from build123d import *

# Parameters (mm, degrees)
SKETCH1_W               = 166
SKETCH1_H               = 116
BOX_SOLID_DEPTH         = 53
BOX_CAVITY_START        = 3
SKETCH2_W               = 160
SKETCH2_H               = 110
BOX_CAVITY_DEPTH        = 53
LID_SCREW_COLUMNS_START = 3
SKETCH3_R               = 3.5
LID_SCREW_COLUMNS_DEPTH = 50
LID_SCREW_HOLES_START   = 53
SKETCH4_R               = 1.25
LID_SCREW_HOLES_DEPTH   = 10
RELAY_BOSSES_START      = 3
SKETCH5_R               = 3.25
RELAY_BOSSES_DEPTH      = 5
RELAY_BOSS_HOLES_START  = 8
SKETCH6_R               = 1.25
RELAY_BOSS_HOLES_DEPTH  = 5
BOARD_PADS_START        = 3
SKETCH7_R               = 2.5
BOARD_PADS_DEPTH        = 5
CABLE_GLAND_HOLES_START = 54
SKETCH8_R               = 6.25
CABLE_GLAND_HOLES_DEPTH = 5
VENT_SLOTS_START        = -84
SKETCH9_W               = 3
SKETCH9_H               = 26
VENT_SLOTS_DEPTH        = 5
SKETCH10_R              = 5
LEG_SOCKETS_DEPTH       = 2


with BuildPart() as part:
    # Sketch1 → Box_Solid (new body)
    with BuildSketch(Plane(origin=(0, 0, 0), x_dir=(1, 0, 0), z_dir=(0, 1, 0))):
        Rectangle(SKETCH1_W, SKETCH1_H)
    extrude(amount=BOX_SOLID_DEPTH)

    # Sketch2 → Box_Cavity (cut)
    with BuildSketch(Plane(origin=(0, 0, 0), x_dir=(1, 0, 0), z_dir=(0, 1, 0)).offset(BOX_CAVITY_START)):
        Rectangle(SKETCH2_W, SKETCH2_H)
    extrude(amount=BOX_CAVITY_DEPTH, mode=Mode.SUBTRACT)

    # Sketch3 → Lid_Screw_Columns (add)
    with BuildSketch(Plane(origin=(0, 0, 0), x_dir=(1, 0, 0), z_dir=(0, 1, 0)).offset(LID_SCREW_COLUMNS_START)):
        with Locations((-77, 52)):
            Circle(SKETCH3_R)
        with Locations((-77, -52)):
            Circle(SKETCH3_R)
        with Locations((77, 52)):
            Circle(SKETCH3_R)
        with Locations((77, -52)):
            Circle(SKETCH3_R)
    extrude(amount=LID_SCREW_COLUMNS_DEPTH)

    # Sketch4 → Lid_Screw_Holes (cut)
    with BuildSketch(Plane(origin=(0, 0, 0), x_dir=(1, 0, 0), z_dir=(0, 1, 0)).offset(LID_SCREW_HOLES_START)):
        with Locations(Location((-77, 52, 0), (0, 0, 270))):
            Circle(SKETCH4_R)
        with Locations(Location((-77, -52, 0), (0, 0, 270))):
            Circle(SKETCH4_R)
        with Locations(Location((77, 52, 0), (0, 0, 270))):
            Circle(SKETCH4_R)
        with Locations(Location((77, -52, 0), (0, 0, 270))):
            Circle(SKETCH4_R)
    extrude(amount=-LID_SCREW_HOLES_DEPTH, mode=Mode.SUBTRACT)

    # Sketch5 → Relay_Bosses (add)
    with BuildSketch(Plane(origin=(0, 0, 0), x_dir=(1, 0, 0), z_dir=(0, 1, 0)).offset(RELAY_BOSSES_START)):
        with Locations(Location((-68.5, 44.5, 0), (0, 0, 90))):
            Circle(SKETCH5_R)
        with Locations(Location((-68.5, -4.5, 0), (0, 0, 90))):
            Circle(SKETCH5_R)
        with Locations(Location((0.5, 44.5, 0), (0, 0, 90))):
            Circle(SKETCH5_R)
        with Locations(Location((0.5, -4.5, 0), (0, 0, 90))):
            Circle(SKETCH5_R)
    extrude(amount=RELAY_BOSSES_DEPTH)

    # Sketch6 → Relay_Boss_Holes (cut)
    with BuildSketch(Plane(origin=(0, 0, 0), x_dir=(1, 0, 0), z_dir=(0, 1, 0)).offset(RELAY_BOSS_HOLES_START)):
        with Locations(Location((-68.5, 44.5, 0), (0, 0, 270))):
            Circle(SKETCH6_R)
        with Locations(Location((-68.5, -4.5, 0), (0, 0, 270))):
            Circle(SKETCH6_R)
        with Locations(Location((0.5, 44.5, 0), (0, 0, 270))):
            Circle(SKETCH6_R)
        with Locations(Location((0.5, -4.5, 0), (0, 0, 270))):
            Circle(SKETCH6_R)
    extrude(amount=-RELAY_BOSS_HOLES_DEPTH, mode=Mode.SUBTRACT)

    # Sketch7 → Board_Pads (add)
    with BuildSketch(Plane(origin=(0, 0, 0), x_dir=(1, 0, 0), z_dir=(0, 1, 0)).offset(BOARD_PADS_START)):
        with Locations(Location((-70.5, -20, 0), (0, 0, 90))):
            Circle(SKETCH7_R)
        with Locations(Location((-70.5, -42, 0), (0, 0, 90))):
            Circle(SKETCH7_R)
        with Locations(Location((-21.5, -20, 0), (0, 0, 90))):
            Circle(SKETCH7_R)
        with Locations(Location((-21.5, -42, 0), (0, 0, 90))):
            Circle(SKETCH7_R)
        with Locations(Location((-12, -32, 0), (0, 0, 90))):
            Circle(SKETCH7_R)
        with Locations(Location((-12, -44, 0), (0, 0, 90))):
            Circle(SKETCH7_R)
        with Locations(Location((10, -32, 0), (0, 0, 90))):
            Circle(SKETCH7_R)
        with Locations(Location((10, -44, 0), (0, 0, 90))):
            Circle(SKETCH7_R)
        with Locations(Location((22, 38, 0), (0, 0, 90))):
            Circle(SKETCH7_R)
        with Locations(Location((22, 12, 0), (0, 0, 90))):
            Circle(SKETCH7_R)
        with Locations(Location((58, 38, 0), (0, 0, 90))):
            Circle(SKETCH7_R)
        with Locations(Location((58, 12, 0), (0, 0, 90))):
            Circle(SKETCH7_R)
        with Locations(Location((22, -8, 0), (0, 0, 90))):
            Circle(SKETCH7_R)
        with Locations(Location((22, -34, 0), (0, 0, 90))):
            Circle(SKETCH7_R)
        with Locations(Location((58, -8, 0), (0, 0, 90))):
            Circle(SKETCH7_R)
        with Locations(Location((58, -34, 0), (0, 0, 90))):
            Circle(SKETCH7_R)
    extrude(amount=BOARD_PADS_DEPTH)

    # Sketch8 → Cable_Gland_Holes (cut)
    with BuildSketch(Plane.XY.offset(CABLE_GLAND_HOLES_START)):
        with Locations(Location((-50, 29.15, 0), (0, 0, 180))):
            Circle(SKETCH8_R)
        with Locations(Location((0, 29.15, 0), (0, 0, 180))):
            Circle(SKETCH8_R)
        with Locations(Location((50, 29.15, 0), (0, 0, 180))):
            Circle(SKETCH8_R)
    extrude(amount=CABLE_GLAND_HOLES_DEPTH, mode=Mode.SUBTRACT)

    # Sketch9 → Vent_Slots (cut)
    with BuildSketch(Plane(origin=(0, 0, 0), x_dir=(0, 0, -1), z_dir=(1, 0, 0)).offset(VENT_SLOTS_START)):
        with Locations((36, 26.5)):
            Rectangle(SKETCH9_W, SKETCH9_H)
        with Locations((24, 26.5)):
            Rectangle(SKETCH9_W, SKETCH9_H)
        with Locations((12, 26.5)):
            Rectangle(SKETCH9_W, SKETCH9_H)
        with Locations((-12, 26.5)):
            Rectangle(SKETCH9_W, SKETCH9_H)
        with Locations((-24, 26.5)):
            Rectangle(SKETCH9_W, SKETCH9_H)
        with Locations((-36, 26.5)):
            Rectangle(SKETCH9_W, SKETCH9_H)
    extrude(amount=VENT_SLOTS_DEPTH, mode=Mode.SUBTRACT)

    # Sketch10 → Leg_Sockets (cut)
    with BuildSketch(Plane(origin=(0, 0, 0), x_dir=(1, 0, 0), z_dir=(0, 1, 0))):
        with Locations(Location((-71, 46, 0), (0, 0, 270))):
            Circle(SKETCH10_R)
        with Locations(Location((-71, -46, 0), (0, 0, 270))):
            Circle(SKETCH10_R)
        with Locations(Location((71, 46, 0), (0, 0, 270))):
            Circle(SKETCH10_R)
        with Locations(Location((71, -46, 0), (0, 0, 270))):
            Circle(SKETCH10_R)
    extrude(amount=LEG_SOCKETS_DEPTH, mode=Mode.SUBTRACT)


solid = part.part
Source: CAD feature listing. Evaluate the final solid. Frame: model axes, mm. A direction names the side the tool comes from. Round coordinates to 2 decimals unless told otherwise and drop trailing zeros. Order: outer loops, then holes, each group sorted by start corner. A loop starts at its lowest first (then second) coordinate and runs counter-clockwise, first axis right, second up. Notation, with made-up numbers: (81, -29) -> (135, -29) arc R11 ccw to (135, -21) -> close; hole circle Ø5 at (16.25, 0.25). An arc over 180 degrees is marked (long way). Answer as CSV lines item,"result".
Item 1: Section C-C, the plane z = 20. Return loops of the section in (x, y).
A:
outline,"(-83, 0) -> (83, 0) -> (83, 53) -> (80, 53) -> (80, 3) -> (-19, 3) -> (-19, 8) -> (-24, 8) -> (-24, 3) -> (-68, 3) -> (-68, 8) -> (-73, 8) -> (-73, 3) -> (-80, 3) -> (-80, 53) -> (-83, 53) -> close"
Item 2: Section B-B, the plane x = -28. Return loops of the section in (y, z).
A:
outline,"(0, -58) -> (53, -58) -> (53, -55) -> (3, -55) -> (3, 55) -> (53, 55) -> (53, 58) -> (0, 58) -> close"
Item 3: Line query: L1, parallel to X at y = 1.2, z = 46; L2, parallel to X at y = 45.25, z = 52; L3, parallel to X at y = 5.95, z = 4.5. Output: solid intervals per line, ascending.
A:
L1,"-83 to -76, -66 to 66, 76 to 83"
L2,"-83 to -78.25, -75.75 to -73.5, 73.5 to 75.75, 78.25 to 83"
L3,"-83 to -80, -71.75 to -69.75, -67.25 to -65.25, -2.75 to -0.75, 1.75 to 3.75, 80 to 83"
Item 4: Pull-direction query (X, two-part tool) for faces 1 (the face through (-1, 0, -1)), 2 (the face through (-23.61, 5.46, 40.66)); classes: pulls with the +X half, pulls with the -X half, needs draft (parallel to the pull), parting line crosses it, or undercut.
A:
face 1,"needs draft"
face 2,"undercut"
Item 5: Section A-A, the plane y = 47.5. Count the separate pieces of the cut face and the enclosed holes in it, plus the area to 3 significant figures.
A:
separate pieces,"1"
enclosed holes,"9"
area,"1,780 mm²"
Item 6: Pin query (flat end, axial travel): pin 1 Ø3 at (x, z) = (-68.5, 4.5) entering from +Y; pin 2 Ø1.2 at (x, z) = (-77, 52) entering from +Y; pin 3 Ø6 at (x, z) = (-62, -37.5) entering from +Y. Return the tip coordinate at first contact, or that it passes through.
A:
pin 1,"y = 8"
pin 2,"y = 43"
pin 3,"y = 3"
Item 7: Reachability of faces 3 (the face through (44.227, 31.544, 56.479)), 4 (the face through (-1, 20, 58)), 5 (the face through (-1, 28, -55)) from +Z, -Z, +X, -X, +Y, -Y: full face, straight path, thin tool, end or side. Return the list, or none.
A:
face 3,"+Z"
face 4,"+Z, +X, -X, +Y, -Y"
face 5,"+Y"
